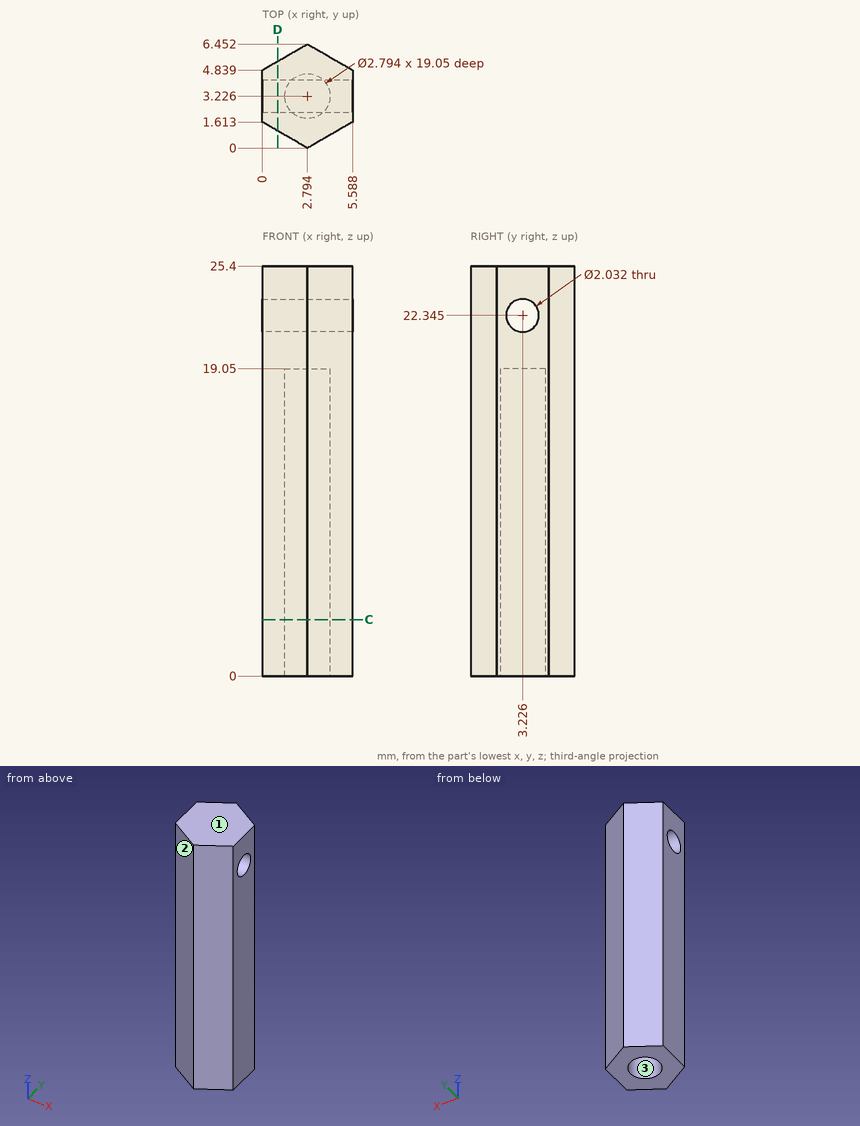
Geometry: see drawing. Coordinates: mm, zero at the bounding-box minimum. Round coordinates to 2 decimals unless told otherwise and drop trailing zeros. Order: outer loops, then holes, each group sorted by start corner. A loop starts at its lowest first (then second) coordinate and runs counter-clockwise, first axis right, second up. Notation, with made-up numbers: (-21.75, -12.5) - (5.25, -12.5) arc R24 ccw to (5.25, 25.5) - close; hole circle Ø1 at (16, 4). An arc over 180 degrees is marked (long way). Use a Markdown table: item, result. Add a question column.
1. Section query D-D (x = 0.95). Return the cut outline in (y, z) (1 decimal).
2. First-contact query: pin 1 (2 mm diameter, centred on x = 2.5, y = 4, fed in from -Z). Flat tip, straight axial feed; report the tip coordinate or a pass-through.
3. Line query: probe 1 along Z at (x, y) = (2.65, 3.25); probe 2 along Y at (x, z) = (2, 17.5) (1 decimal); probe 3 along Y at (x, z) = (3.45, 12.25) (1 decimal). Output: solid intervals per line, ascending.
4. Mould query, pull axis Y, two halves, no side actions, for the marked faces 1, 2 and 3. Classes: +Y half, -Y half, draft (parallel to the pull), parting line (faces both ways), or undercut.
5. Section query C-C (z = 3.5). Return the cut outline in (x, y), then the cut area to 3 significant figures.
Derived:
| question | item | result |
|---|---|---|
| 1 | outline | (1.1, 0) - (5.4, 0) - (5.4, 25.4) - (1.1, 25.4) - close; hole circle Ø2 at (3.2, 22.3) |
| 2 | pin 1 | z = 0 |
| 3 | probe 1 | 19.05 to 21.33, 23.36 to 25.4 |
| 3 | probe 2 | 0.5 to 2.1, 4.4 to 6 |
| 3 | probe 3 | 0.4 to 2, 4.5 to 6.1 |
| 4 | face 1 | draft |
| 4 | face 2 | -Y half |
| 4 | face 3 | undercut |
| 5 | outline | (0, 1.61) - (2.79, 0) - (5.59, 1.61) - (5.59, 4.84) - (2.79, 6.45) - (0, 4.84) - close; hole circle Ø2.79 at (2.79, 3.23) |
| 5 | area | 20.9 mm2 |
